Input: part model. Units: mm. Frame: model coordinates. Face numbers are marked on the shaded views. A direction names the side the tool comes from. Coordinates: 2 decimals unless noted, no trailing zeros. Order: outer loops, then holes, each group sorted by start corner. A loop starts at its lowest first (then second) coordinate and runs counter-clockwise, first axis right, second up. Notation, with made-up numbers: (-18, 25.5) -> (21, 25.5) arc R21 ccw to (21, 39.5) -> close; hole circle Ø3 at (-24, 64.5). An arc over 180 degrees is marked (long way). Write each question's results on one line, items separated by ' | '.
```python
from build123d import *

# Parameters (mm, degrees)
RESSALTO_EXTRUS_O1_DEPTH                    = 60
RESSALTO_EXTRUS_O2_DEPTH                    = 4
RESSALTO_EXTRUS_O3_DEPTH                    = 4
FURO_ROSCADO_PARA_CONDU_TE_DE_M3X0_51_D     = 3.15
FURO_ROSCADO_PARA_CONDU_TE_DE_M3X0_51_DEPTH = 10
FURO_ROSCADO_PARA_CONDU_TE_DE_M3X0_51_TIP   = 0.946355475
FURO_ROSCADO_PARA_CONDU_TE_DE_M3X0_52_D     = 3.15
FURO_ROSCADO_PARA_CONDU_TE_DE_M3X0_52_DEPTH = 7.5
FURO_ROSCADO_PARA_CONDU_TE_DE_M3X0_52_TIP   = 0.946355475
FILETE1_R                                   = 1
FILETE2_R                                   = 5


with BuildPart() as part:
    # Esboço1 → Ressalto-extrusão1 (new body)
    with BuildSketch(Plane.XY):
        Polygon((0, 0), (18, 0), (0, 18), align=None)
    extrude(amount=RESSALTO_EXTRUS_O1_DEPTH)

    # Esboço2 → Ressalto-extrusão2 (add)
    with BuildSketch(Plane.XY.offset(60)):
        Polygon((0, 0), (0, 5), (5, 0), align=None)
    extrude(amount=RESSALTO_EXTRUS_O2_DEPTH)

    # Esboço3 → Ressalto-extrusão3 (add)
    with BuildSketch(Plane(origin=(0, 0, 0), x_dir=(-1, 0, 0), z_dir=(0, 0, -1))):
        Polygon((0, 0), (0, 5), (-5, 0), align=None)
    extrude(amount=RESSALTO_EXTRUS_O3_DEPTH)

    # Furo roscado para conduíte de M3x0.51
    with Locations(Plane.XY.offset(60)):
        with Locations((7, 5)):
            Hole(FURO_ROSCADO_PARA_CONDU_TE_DE_M3X0_51_D / 2, depth=FURO_ROSCADO_PARA_CONDU_TE_DE_M3X0_51_DEPTH)
            with Locations((0, 0, -(FURO_ROSCADO_PARA_CONDU_TE_DE_M3X0_51_DEPTH + FURO_ROSCADO_PARA_CONDU_TE_DE_M3X0_51_TIP / 2))):  # 118° drill point
                Cone(0, FURO_ROSCADO_PARA_CONDU_TE_DE_M3X0_51_D / 2, FURO_ROSCADO_PARA_CONDU_TE_DE_M3X0_51_TIP, mode=Mode.SUBTRACT)

    # Furo roscado para conduíte de M3x0.52
    with Locations(Plane(origin=(0, 0, 0), x_dir=(-1, 0, 0), z_dir=(0, 0, -1))):
        with Locations((-7, 5)):
            Hole(FURO_ROSCADO_PARA_CONDU_TE_DE_M3X0_52_D / 2, depth=FURO_ROSCADO_PARA_CONDU_TE_DE_M3X0_52_DEPTH)
            with Locations((0, 0, -(FURO_ROSCADO_PARA_CONDU_TE_DE_M3X0_52_DEPTH + FURO_ROSCADO_PARA_CONDU_TE_DE_M3X0_52_TIP / 2))):  # 118° drill point
                Cone(0, FURO_ROSCADO_PARA_CONDU_TE_DE_M3X0_52_D / 2, FURO_ROSCADO_PARA_CONDU_TE_DE_M3X0_52_TIP, mode=Mode.SUBTRACT)

    # Filete1
    filete1_edges = [part.edges().sort_by_distance(p)[0] for p in [
        (18, 0, 30),
    ]]
    fillet(filete1_edges, radius=FILETE1_R)

    # Filete2
    filete2_edges = [part.edges().sort_by_distance(p)[0] for p in [
        (0, 18, 30),
    ]]
    fillet(filete2_edges, radius=FILETE2_R)


solid = part.part
```
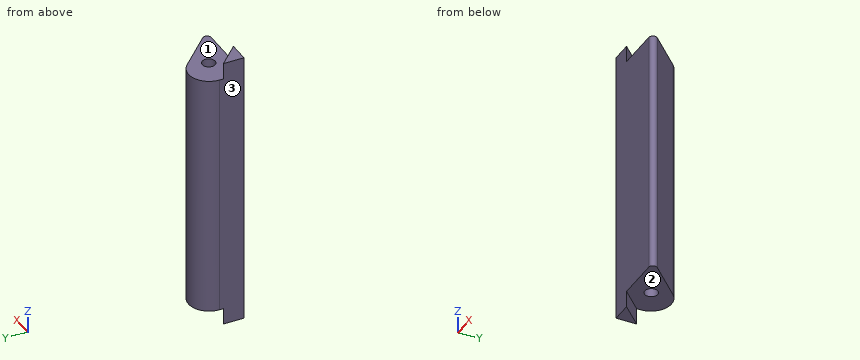
(1) Cut plane B-B, the plane x = 3.25. Return loops of the section in (y, z).
Return value:
outline: (0, -4) -> (1.75, -4) -> (1.75, 0) -> (10.61, 0) -> (10.61, 60) -> (1.75, 60) -> (1.75, 64) -> (0, 64) -> close
(2) Reachability of the marked faces 1, 2 and 3 from +Z, -Z, +X, -X, +Y, -Y: full face, straight path, thin tool, end or side. Return the list, or none.
Return value:
face 1: +Z, +X, +Y | face 2: -Z, +X, +Y | face 3: +Z, -Z, -X, +Y, -Y
(3) Line query: line 1 along Z through (x, y) = (7.25, 7.25); line 2 along Y through (x, z) = (7, 4.25) (1 decimal); line 3 along X through (y, z) = (5, 54.75) (3 decimals). Output: solid intervals per line, ascending. Write a range as from..to.
Return value:
line 1: 0..60 | line 2: 0..3.4, 6.6..10.5 | line 3: 0..5.425, 8.575..13
(4) Cut plane D-D, the plane x = 13.5. Return loops of the section in (y, z), plus the area to 3 significant figures.
Return value:
outline: (0, 0) -> (4.5, 0) -> (4.5, 60) -> (0, 60) -> close | area: 270 mm2
(5) Cut plane C-C, the plane z = 28.5. Return loops of the section in (x, y).
Return value:
outline: (0, 0) -> (15.59, 0) arc R1 ccw to (16.29, 1.71) -> (8.54, 9.46) arc R5 ccw to (0, 5.93) -> close
(6) Pin query (flat end, axial travel): P1, Ø6, axis at x = 3.5, y = 2, coming from the -Z side; P2, Ø1.5, axis at x = 14.5, z = 10.5, coming from the +Y side; P3, Ø5, axis at x = 7, y = 5, coming from the +Z side; P4, Ø3, axis at x = 10.5, z = 27, coming from the +Y side. Return the tip coordinate at first contact, or that it passes through.
Return value:
P1: z = -4 | P2: y = 4.25 | P3: z = 60 | P4: y = 9
(7) Cut plane A-A, the plane z = 1. Return loops of the section in (x, y) (3 decimals), plus the area to 3 significant figures.
Return value:
outline: (0, 0) -> (15.586, 0) arc R1 ccw to (16.293, 1.707) -> (8.536, 9.464) arc R5 ccw to (0, 5.929) -> close; hole circle Ø3.15 at (7, 5) | area: 122 mm2
